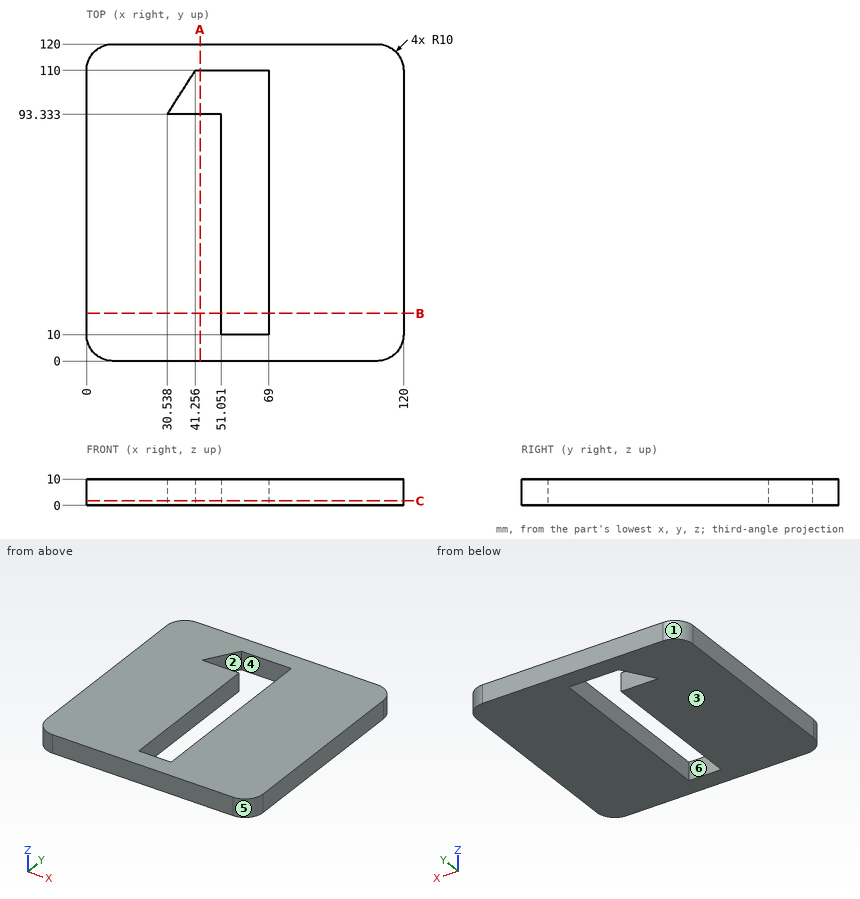
Study the drawing (mm; zero at the part's minimum x, y, z) and answer. A direction names the side the tool comes from. Coordinates: 2 decimals unless noted, no trailing zeros. Write each loop counter-clockwise with the first axis right and the second up, starting at its lowest first coordinate (ties: lowest second). Pieces come first, ordered by that corner, then holes. Notation, with made-up numbers: (-23, -21) - (-8, -21) arc R12 cw to (-8, -9) - close; hole circle Ø4 at (34.5, 50.5). An arc over 180 degrees is marked (long way). Answer as a JSON object with one key per item and string values.
Q1. Find section C-C (z = 1.75). Write down the section's boundary in (x, y) (1 decimal), plus the area to 3 significant figures.
Results list:
{"outline": "(0, 10) arc R10 ccw to (10, 0) - (110, 0) arc R10 ccw to (120, 10) - (120, 110) arc R10 ccw to (110, 120) - (10, 120) arc R10 ccw to (0, 110) - close; hole (30.5, 93.3) - (51.1, 93.3) - (51.1, 10) - (69, 10) - (69, 110) - (41.3, 110) - close", "area": "12,300 mm^2"}
Q2. Which of the six approach directions +Z, -Z, +X, -X, +Y, -Y give full straight-line access (tool end or side, diameter ignored) to the marked faces 5 and 6?
Results list:
{"face 5": "+Z, -Z, +X, -Y", "face 6": "+Z, -Z"}
Q3. For a pull along X with two mould halves and no side action, classify the marked faces 1, 2, 3 and 4 as pulls with the +X half, pulls with the -X half, needs draft (parallel to the pull), parting line crosses it, or undercut.
Results list:
{"face 1": "pulls with the -X half", "face 2": "undercut", "face 3": "needs draft", "face 4": "undercut"}
Q4. Given pin 1 Ø1 at (x, y) = (36.5, 69.5) entering from -Z; pin 2 Ø8 at (x, y) = (56, 47) entering from -Z, each flat-ended and moving along its own axis, determine where each tip first touches the part or whether it passes through.
Results list:
{"pin 1": "stops at z = 0", "pin 2": "passes through"}
Q5. Find section A-A (x = 43). Write down the section's boundary in (y, z), plus the area to 3 significant figures.
Results list:
{"outline": "(0, 0) - (93.33, 0) - (93.33, 10) - (0, 10) - close; (110, 0) - (120, 0) - (120, 10) - (110, 10) - close", "area": "1,030 mm^2"}
Q6. Consider L1, parallel to X at y = 22.5, z = 5; L2, parallel to X at y = 100, z = 2 (1 decimal); L3, parallel to X at y = 8, z = 6.25. Determine where each line is inside the solid, lowest interval first. Write a range as from..to.
Results list:
{"L1": "x = 0..51.05, 69..120", "L2": "x = 0..34.8, 69..120", "L3": "x = 0.2..119.8"}
Q7. Find section B-B (y = 18). Write down the section's boundary in (x, z), plus the area to 3 significant figures.
Results list:
{"outline": "(0, 0) - (51.05, 0) - (51.05, 10) - (0, 10) - close; (69, 0) - (120, 0) - (120, 10) - (69, 10) - close", "area": "1,020 mm^2"}
